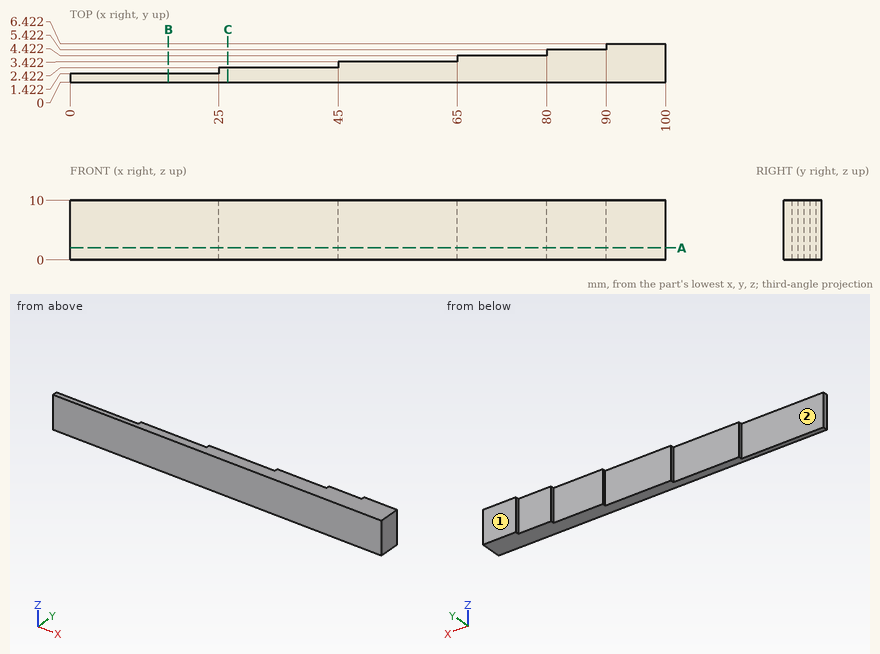
Geometry check sheet. Reference: drawing and pictorial views, mm from the part's lowest x, y, z. A direction names the side the tool comes from. Coordinates: 2 decimals unless noted, no trailing zeros. Write each loop counter-clockwise with the first axis right and the second up, starting at its lowest first coordinate (ties: lowest second). Pieces come first, ordered by that corner, then holes. Notation, with made-up numbers: (22.25, 46) - (55.25, 46) arc R18 ccw to (55.25, 54) - close; hole circle Ø9 at (3.5, 75). An arc over 180 degrees is marked (long way). Write item = value, one per line.
Q1. Cross-section at A-A (z = 2). Enter the section's corners in (x, y), plus the area to 3 significant figures.
Answer:
outline = (0, 0) - (100, 0) - (100, 6.42) - (90, 6.42) - (90, 5.42) - (80, 5.42) - (80, 4.42) - (65, 4.42) - (65, 3.42) - (45, 3.42) - (45, 2.42) - (25, 2.42) - (25, 1.42) - (0, 1.42) - close
area = 337 mm²
Q2. Cross-section at C-C (x = 26.5). Enter the section's corners in (y, z).
Answer:
outline = (0, 0) - (2.42, 0) - (2.42, 10) - (0, 10) - close
Q3. Material ranges on L1, parallel to Y at x = 74, z = 5.75; L2, parallel to Y at x = 48, z = 1.25; L3, parallel to X at y = 2.25, z = 9.5, recorded low to high. Write a range as from..to.
Answer:
L1 = 0..4.42
L2 = 0..3.42
L3 = 25..100
Q4. Go/stop test with flat-tipped pins: pin 1 Ø0.5 at (y, z) = (6, 4.5) entering from -X; pin 2 Ø3 at (x, z) = (75.5, 6) entering from +Y; pin 3 Ø3 at (x, z) = (56, 3) entering from +Y. Record where each tip stops, or that it passes through.
Answer:
pin_1 = 90
pin_2 = 4.42
pin_3 = 3.42
Q5. Cross-section at B-B (x = 16.5). Enter the section's corners in (y, z), plus the area to 3 significant figures.
Answer:
outline = (0, 0) - (1.42, 0) - (1.42, 10) - (0, 10) - close
area = 14.2 mm²
Q6. Access from +Z, -Z, +X, -X, +Y, -Y to the whole of each face (thin tool, end or side, straight path). Record for the marked faces 1 and 2.
Answer:
face_1 = +Z, -Z, +X, -X, +Y
face_2 = +Z, -Z, -X, +Y
